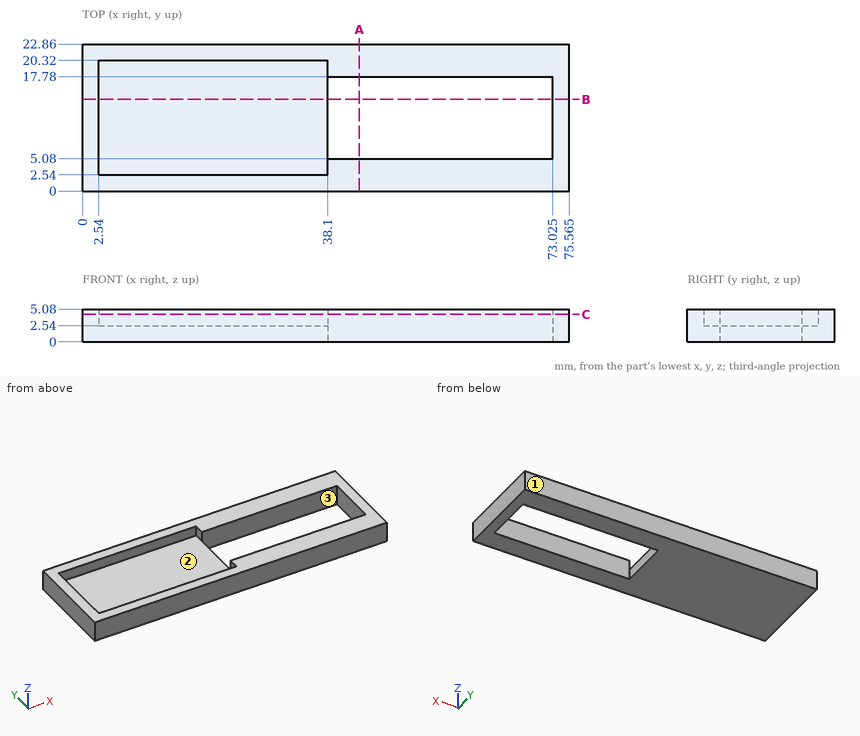
Study the drawing (mm; zero at the part's minimum x, y, z) and answer. A direction names the side the tool comes from. Round coordinates to 2 decimals unless told otherwise and drop trailing zeros. Loops run counter-clockwise (first coordinate to the right, second up) from the corner with the lowest first, then second, coordinate; pieces in that order, holes last.
Q1. Section A-A, the plane x = 43 is taken. Determine the outline of the cut face in (y, z).
Q2. Given pin 1 Ø1.5 at (x, y) = (26, 5.5) entering from -Z; pin 2 Ø1 at (x, y) = (53, 16) entering from -Z; pin 3 Ø12 at (x, y) = (32.5, 11.5) entering from +Z, each flat-ended and moving along its own axis, determine where each tip first touches the part or whether it passes through.
Q3. Find the intervals of material crossed by line 1 (X direction, y = 12.75, z = 4.8) (3 decimals); line 2 (Y direction, x = 17, z = 3.95); line 3 (X direction, y = 14.5, z = 1.65) (3 decimals), in increasing order.
Q4. Which of the six approach directions +Z, -Z, +X, -X, +Y, -Y give full straight-line access (tool end or side, diameter ignored) to the marked faces 1, 2 and 3?
Q5. Section B-B, the plane y = 14.25 is taken. Determine the outline of the cut face in (x, z) (3 decimals).
Q6. Section C-C, the plane z = 4.3 is taken. Determine the outline of the cut face in (x, y) (3 decimals), then the cut area to 3 significant figures.
Completed:
1. outline: (0, 0) - (5.08, 0) - (5.08, 5.08) - (0, 5.08) - close; (17.78, 0) - (22.86, 0) - (22.86, 5.08) - (17.78, 5.08) - close
2. pin 1: stops at z = 0
2. pin 2: passes through
2. pin 3: stops at z = 2.54
3. line 1: x = 0 to 2.54, 73.025 to 75.565
3. line 2: y = 0 to 2.54, 20.32 to 22.86
3. line 3: x = 0 to 38.1, 73.025 to 75.565
4. face 1: +Z, -Z, +X, -X, +Y
4. face 2: +Z
4. face 3: +Z, -Z
5. outline: (0, 0) - (38.1, 0) - (38.1, 2.54) - (2.54, 2.54) - (2.54, 5.08) - (0, 5.08) - close; (73.025, 0) - (75.565, 0) - (75.565, 5.08) - (73.025, 5.08) - close
6. outline: (0, 0) - (75.565, 0) - (75.565, 22.86) - (0, 22.86) - close; hole (2.54, 2.54) - (38.1, 2.54) - (38.1, 5.08) - (73.025, 5.08) - (73.025, 17.78) - (38.1, 17.78) - (38.1, 20.32) - (2.54, 20.32) - close
6. area: 652 mm2
